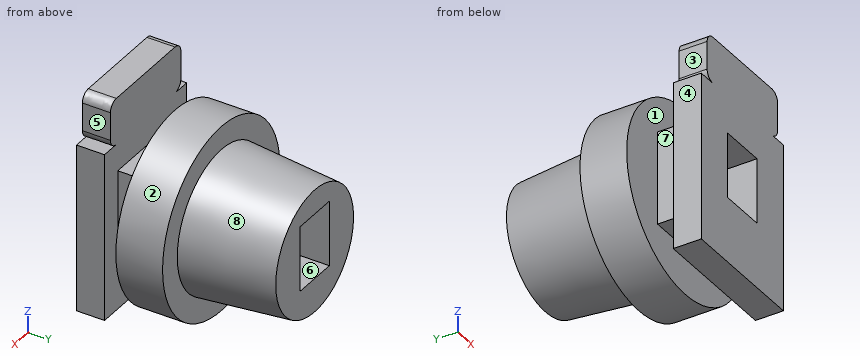
Autodesk Inventor part; units mm, degrees
ref_plane "YZ Plane" through (0, 0, 0) normal (1, 0, 0) x (0, 1, 0)
ref_plane "XZ Plane" through (0, 0, 0) normal (0, 1, 0) x (-1, 0, 0)
ref_plane "XY Plane" through (0, 0, 0) normal (0, 0, 1) x (1, 0, 0)
sketch "Sketch3" plane through (0, 0, 0) normal (0, 1, 0) x (-1, 0, 0)
  spline S0 degree 3 poles (2.0049, 23.0048) (1.4509, 23.0048) (1.005, 22.5589) (1.005, 22.0049) knots 0 0 0 0 1 1 1 1
  line L0 (2.0049, 23.0048) -> (1.4509, 23.0048) construction
  line L1 (1.4509, 23.0048) -> (1.005, 22.5589) construction
  line L2 (1.005, 22.5589) -> (1.005, 22.0049) construction
  spline S1 degree 3 poles (1.005, 19.0051) (1.005, 18.4511) (1.4509, 18.0046) (2.0049, 18.0046) knots 0 0 0 0 1 1 1 1
  line L3 (1.005, 19.0051) -> (1.005, 18.4511) construction
  line L4 (1.005, 18.4511) -> (1.4509, 18.0046) construction
  line L5 (1.4509, 18.0046) -> (2.0049, 18.0046) construction
  line L6 (1.005, 22.0049) -> (1.005, 19.0051)
  spline S2 degree 3 poles (12.0053, 18.0046) (12.5593, 18.0046) (13.0053, 18.4511) (13.0053, 19.0051) knots 0 0 0 0 1 1 1 1
  line L7 (12.0053, 18.0046) -> (12.5593, 18.0046) construction
  line L8 (12.5593, 18.0046) -> (13.0053, 18.4511) construction
  line L9 (13.0053, 18.4511) -> (13.0053, 19.0051) construction
  line L10 (2.0049, 18.0046) -> (0.005, 18.0046)
  line L11 (0.005, 18.0046) -> (0.005, 0.0047)
  line L12 (0.005, 0.0047) -> (14.0052, 0.0048)
  line L13 (14.0052, 0.0048) -> (14.0052, 18.0046)
  line L14 (14.0052, 18.0046) -> (12.0053, 18.0046)
  spline S3 degree 3 poles (13.0053, 22.0049) (13.0053, 22.5589) (12.5593, 23.0048) (12.0053, 23.0048) knots 0 0 0 0 1 1 1 1
  line L15 (13.0053, 22.0049) -> (13.0053, 22.5589) construction
  line L16 (13.0053, 22.5589) -> (12.5593, 23.0048) construction
  line L17 (12.5593, 23.0048) -> (12.0053, 23.0048) construction
  line L18 (13.0053, 19.0051) -> (13.0053, 22.0049)
  line L19 (12.0053, 23.0048) -> (2.0049, 23.0048)
  point P0 (0, 0)
  point P1 (2.0049, 23.0048)
  point P2 (1.005, 22.0049)
  point P3 (1.005, 19.0051)
  point P4 (2.0049, 18.0046)
  point P5 (0.005, 18.0046)
  point P6 (12.0054, 18.0046)
  point P7 (12.0053, 23.0048)
extrude "Extrusion2" add sketch "Sketch3" along normal blind 3
ref_plane "Edge of module" through (0, 6.1, 0) normal (0, 1, 0) x (1, 0, 0)
sketch "Sketch5" plane through (0, 3, 0) normal (0, 1, 0) x (1, 0, 0)
  line L0 (-0.005, -18.0046) -> (-0.005, -0.0047)
  line L1 (-0.005, -3.5047) -> (-14.0052, -3.5048) construction
  line L2 (-14.0052, -0.0048) -> (-14.0052, -18.0046)
  line L3 (-0.005, -0.0047) -> (-14.0052, -0.0048)
  line L4 (-0.005, -0.0047) -> (-14.0052, -0.0048) construction
  line L5 (-7.0051, -0.0047) -> (-7.0051, -23.0048) construction
  line L6 (-12.0053, -23.0048) -> (-2.0049, -23.0048) construction
  line L7 (-2.2551, -15.0047) -> (-2.2551, -5.0047)
  line L8 (-2.2551, -5.0047) -> (-11.7551, -5.0047)
  line L9 (-11.7551, -5.0047) -> (-11.7551, -15.0047)
  line L10 (-11.7551, -15.0047) -> (-2.2551, -15.0047)
  line L11 (-2.2551, -15.0047) -> (-11.7551, -5.0047) construction
  line L12 (-2.2551, -5.0047) -> (-11.7551, -15.0047) construction
  point P0 (0, 0)
  point P1 (-7.0051, -10.0047)
  dimension "d9" = 3.5
  dimension "d10" = 9.5
  dimension "d11" = 10
  dimension "d12" = 1.5
extrude "Extrusion3" add sketch "Sketch5" along normal up to surface (3.1 mm away)
sketch "Sketch6" plane through (-11.7551, 6.1, 5.0047) normal (0, 1, 0) x (1, 0, 0)
  line L0 (4.75, 5) -> (4.75, -18.0001) construction
  line L1 (9.5, -10) -> (0, -10) construction
  line L2 (9.5, -10) -> (0, 0) construction
  circle A0 centre (4.75, -5) radius 10
  point P0 (11.7551, 5.0047)
  dimension "d15" = 20
extrude "Extrusion4" add sketch "Sketch6" along normal blind 5
sketch "Sketch7" plane through (-7.0051, 11.1, 10.0047) normal (0, 1, 0) x (1, 0, 0)
  circle A0 centre (0, 0) radius 7.5
  point P0 (7.0051, 10.0047)
  dimension "d18" = 15
extrude "Extrusion5" add sketch "Sketch7" along normal blind 10 draft -5
ref_plane "Work Plane5" through (-0.005, 0, 0.0047) normal (0, 0, -1) x (-1, 0, 0)
sketch "Sketch8" plane through (0, 0, 0) normal (0, -1, 0) x (1, 0, 0)
  line L0 (-9.5051, 7.0047) -> (-4.5051, 7.0047)
  line L1 (-4.5051, 7.0047) -> (-4.5051, 14.0047)
  line L2 (-4.5051, 14.0047) -> (-9.5051, 14.0047)
  line L3 (-9.5051, 14.0047) -> (-9.5051, 7.0047)
  line L4 (-9.5051, 7.0047) -> (-4.5051, 14.0047) construction
  line L5 (-4.5051, 7.0047) -> (-9.5051, 14.0047) construction
  line L6 (-0.005, 0.0047) -> (-14.0052, 0.0048) construction
  line L7 (-7.0051, 0.0047) -> (-7.0051, 22.9634) construction
  line L8 (2.801, 0.0047) -> (-16.8063, 0.0048)
  point P0 (0, 0)
  point P1 (-7.0051, 10.5047)
  dimension "d21" = 5
  dimension "d22" = 7
  dimension "d24" = 7
extrude "Extrusion6" cut sketch "Sketch8" against normal through all
properties part number "Ant connector"
Verification items for the finished model (mm, model axes). Face numbers are marked on the shaded views. A direction names the side the tool comes from. Give positions to 0.01 mm unless a question says otherwise; leave off trailing zeros. Write each loop counter-clockwise with the first axis right and the second up, starting at its lowest first coordinate (ties: lowest second). Pieces come first, ordered by that corner, then holes. Notation, with made-up numbers: M 47,12.25 L 103,12.25 A15 ccw 103,33.25 Z; hole C 38.5,0.5 d1. An arc over 180 degrees is marked long. Use CSV: the item, a comma, the result in double quotes.
1) Cross-section at B-B (y = 4.5). Enter the section's corners in (x, z).
Final values:
outline,"M -11.76,5 L -2.26,5 L -2.26,15 L -11.76,15 Z; hole M -9.51,7 L -4.51,7 L -4.51,14 L -9.51,14 Z"
2) Go/stop test with flat-tipped pins: pin 1 Ø2.5 at (y, z) = (1, 21) entering from -X; pin 2 Ø8 at (y, z) = (16, 19.5) entering from -X; pin 3 Ø8 at (y, z) = (14.5, 5) entering from -X. Record where each tip stops, or that it passes through.
Final values:
pin 1,"x = -13.01"
pin 2,"x = -11.49"
pin 3,"x = -16.58"
3) Access from +Z, -Z, +X, -X, +Y, -Y to the whole of each face (thin tool, end or side, straight path). Record for the marked faces 1, 2, 3, 4 and 5.
Final values:
face 1,"none"
face 2,"+Y"
face 3,"+Z, -X, +Y, -Y"
face 4,"+Z, -Z, -X, -Y"
face 5,"+Z, +X, +Y, -Y"
4) Cross-section at C-C (x = -1.5). State how many separate pieces and enclosed holes the cut face has, plus the area to 3 significant figures.
Final values:
separate pieces,"3"
enclosed holes,"0"
area,"240 mm²"
5) Material ranges on line 1 along Z through (x, y) = (-7, 8.75); line 2 along Z through (x, y) = (-4.75, 1.75); line 3 along Y through (x, z) = (-1.25, 12.75), recorded low to high.
Final values:
line 1,"0 to 7, 14 to 20"
line 2,"0 to 7, 14 to 23"
line 3,"0 to 3, 6.1 to 21.1"
6) Release check for a two-part mould opening along Z. For the marked faces 6, 7 and 8 record: released by +Z, released by -Z, zero draft, split by the parting line, or undercut.
Final values:
face 6,"undercut"
face 7,"zero draft"
face 8,"split by the parting line"
7) Cross-section at A-A (z = 1.5). Enter the section's corners in (x, y) (3 decimals).
Final values:
outline,"M -14.005,0 L -0.005,0 L -0.005,3 L -14.005,3 Z; M -12.265,6.1 L -1.745,6.1 L -1.745,11.1 L -12.265,11.1 Z"
8) Cross-section at D-D (y = 10.25). Enter the section's corners in (x, z), plus the area to 3 significant figures.
Final values:
outline,"C -7.01,10 d20; hole M -9.51,7 L -4.51,7 L -4.51,14 L -9.51,14 Z"
area,"279 mm²"
